Geometry: final body of the model. Coordinates: model frame, mm. A direction names the side the tool comes from. Coordinates: 2 decimals unless noted, no trailing zeros. Write each loop counter-clockwise with the first axis right and the second up, starting at its lowest first coordinate (ties: lowest second). Pieces come first, ordered by that corner, then holes.
from build123d import *

# Parameters (mm, degrees)
F1_DEPTH = 25.4


with BuildPart() as f1:
    # F0 (on Front) → F1 (new body)
    with BuildSketch(Plane.XZ):
        with BuildLine():
            add(Edge.make_bspline(
                [(-33.719659, 5.282047), (-28.87602, 13.115586), (-24.032382, 20.949125), (-19.188743, 28.782664)],
                knots=[0, 0, 0, 0, 27.630174, 27.630174, 27.630174, 27.630174], degree=3))
            Line((-33.719659, 5.282047), (-38.055241, 5.303812))
            Line((-38.055241, 5.303812), (-38.055241, -7.445157))
            Line((-38.055241, -7.445157), (-13.75252, -7.445157))
            Line((-13.75252, -7.445157), (-13.75252, 5.303812))
            Line((-13.75252, 5.303812), (-17.565828, 5.303812))
            Line((-17.565828, 5.303812), (-9.939212, 16.686819))
            Line((-9.939212, 16.686819), (-7.91495, 13.499577))
            Line((-7.91495, 13.499577), (-10.280703, 13.499577))
            Line((-10.280703, 13.499577), (-10.280703, 0))
            Line((-10.280703, 0), (17.152347, 0))
            Line((17.152347, 0), (17.152347, 13.499577))
            Line((17.152347, 13.499577), (15.103405, 13.499577))
            Line((15.103405, 13.499577), (17.152347, 16.686819))
            Line((17.152347, 16.686819), (24.20981, 4.962322))
            Line((24.20981, 4.962322), (20.681079, 4.962322))
            Line((20.681079, 4.962322), (20.681079, -7.331326))
            Line((20.681079, -7.331326), (45.609865, -7.331326))
            Line((45.609865, -7.331326), (45.609865, 5.303812))
            Line((45.609865, 5.303812), (40.601343, 5.303812))
            Line((40.601343, 5.303812), (25.6896, 28.782664))
            Line((25.6896, 28.782664), (29.218335, 28.782664))
            Line((29.218335, 28.782664), (29.218335, 41.729435))
            Line((29.218335, 41.729435), (5.086357, 41.729435))
            Line((5.086357, 41.729435), (5.086357, 28.782664))
            Line((5.086357, 28.782664), (8.273601, 28.782664))
            add(Edge.make_bspline(
                [(3.378906, 21.467682), (5.010471, 23.906009), (6.642036, 26.344337), (8.273601, 28.782664)],
                knots=[0, 0, 0, 0, 8.801534, 8.801534, 8.801534, 8.801534], degree=3))
            add(Edge.make_bspline(
                [(-1.288126, 28.782664), (0.267551, 26.344337), (1.823229, 23.906009), (3.378906, 21.467682)],
                knots=[0, 0, 0, 0, 8.67699, 8.67699, 8.67699, 8.67699], degree=3))
            add(Edge.make_bspline(
                [(1.899114, 28.782664), (0.836701, 28.782664), (-0.225713, 28.782664), (-1.288126, 28.782664)],
                knots=[0, 0, 0, 0, 3.18724, 3.18724, 3.18724, 3.18724], degree=3))
            add(Edge.make_bspline(
                [(1.899114, 41.729435), (1.899114, 37.413845), (1.899114, 33.098254), (1.899114, 28.782664)],
                knots=[0, 0, 0, 0, 12.946771, 12.946771, 12.946771, 12.946771], degree=3))
            add(Edge.make_bspline(
                [(-22.23286, 41.729435), (-14.188869, 41.729435), (-6.144877, 41.729435), (1.899114, 41.729435)],
                knots=[0, 0, 0, 0, 24.131975, 24.131975, 24.131975, 24.131975], degree=3))
            add(Edge.make_bspline(
                [(-22.23286, 28.782664), (-22.23286, 33.098254), (-22.23286, 37.413845), (-22.23286, 41.729435)],
                knots=[0, 0, 0, 0, 12.946771, 12.946771, 12.946771, 12.946771], degree=3))
            add(Edge.make_bspline(
                [(-19.188743, 28.782664), (-20.203449, 28.782664), (-21.218155, 28.782664), (-22.23286, 28.782664)],
                knots=[0, 0, 0, 0, 3.044117, 3.044117, 3.044117, 3.044117], degree=3))
        make_face()
    extrude(amount=F1_DEPTH)


solid = f1.part
Item 1: Set-up query: faces 1 (the flat face through (17.152, -13, 7)), 2 (the flat face through (29.218, -13, 35)), 3 (the flat face through (33.25, -12.52, 16.88)). Return all of +Z, -Z, +X, -X, +Y, -Y with unobstructed straight access to the full face (end or side cutting, diameter ignored); none if empty.
Derived:
face 1: -Z, +Y, -Y
face 2: +Z, +X, +Y, -Y
face 3: +X, +Y, -Y
Item 2: Pin query (flat end, axial travel): pin 1 (7.5 mm diameter, centred on x = 10.5, y = -11, fed in from -Z); pin 2 (1 mm diameter, centred on x = 19.5, z = 24, fed in from +Y); pin 3 (2 mm diameter, centred on y = -21.5, z = 22, fed in from -X); pin 4 (10.5 mm diameter, centred on y = -17, z = 34.5, fed in from -X). Return the tip coordinate at first contact, or that it passes through.
Derived:
pin 1: stops at z = 0
pin 2: stops at y = 0
pin 3: stops at x = -24
pin 4: stops at x = -22.23
Item 3: Pull-direction query (X, two-part tool) for faces 4 (the flat face through (16, -13, 13.5)), 5 (the flat face through (-38.055, -13, -1)), 6 (the flat face through (33, -13, -7.331)); classes: released by +X, released by -X, zero draft, split by the parting line, or undercut.
Derived:
face 4: undercut
face 5: released by -X
face 6: zero draft
Item 4: Section B-B, the plane z = -4. Output: boundary loops of the cut face in (x, y).
Derived:
outline: (-38.06, -25.4) - (-13.75, -25.4) - (-13.75, 0) - (-38.06, 0) - close; (20.68, -25.4) - (45.61, -25.4) - (45.61, 0) - (20.68, 0) - close
Item 5: Section A-A, the plane z = 4. Output: boundary loops of the cut face in (x, y).
Derived:
outline: (-38.06, -25.4) - (-13.75, -25.4) - (-13.75, 0) - (-38.06, 0) - close; (-10.28, -25.4) - (17.15, -25.4) - (17.15, 0) - (-10.28, 0) - close; (20.68, -25.4) - (45.61, -25.4) - (45.61, 0) - (20.68, 0) - close
Item 6: Section C-C, the plane x = 12. Output: boundary loops of the cut face in (y, z).
Derived:
outline: (-25.4, 0) - (0, 0) - (0, 41.73) - (-25.4, 41.73) - close
Item 7: Material intervals for probe 1 along X at (y, z) = (-16.5, 2.5); probe 2 along X at (y, z) = (-8.5, 31); probe 3 along X at (y, z) = (-2.75, 10.5), sorted ascending.
Derived:
probe 1: x = -38.06 to -13.75, -10.28 to 17.15, 20.68 to 45.61
probe 2: x = -22.23 to 1.9, 5.09 to 29.22
probe 3: x = -30.49 to -14.08, -10.28 to 17.15, 20.88 to 37.3
